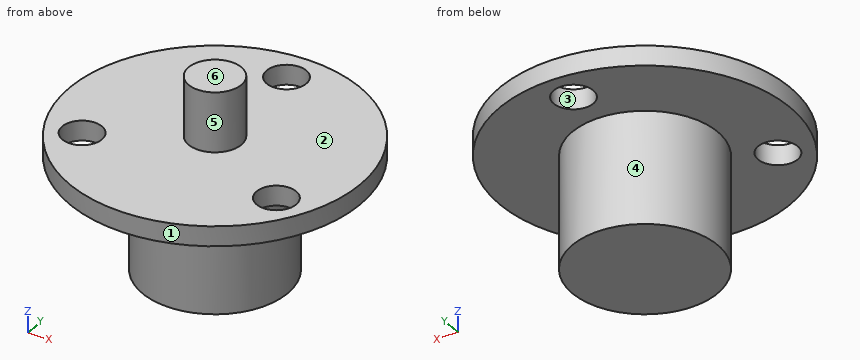
from build123d import *

# Parameters (mm, degrees)
ESQUISSE1_R             = 11
BOSS_EXTRU_1_DEPTH      = 17
ESQUISSE2_R             = 22
BOSS_EXTRU_2_DEPTH      = 3
ESQUISSE3_R             = 4
BOSS_EXTRU_3_DEPTH      = 9
ENL_V_MAT_EXTRU_1_REACH = 38.986
ESQUISSE5_R             = 3


with BuildPart() as part:
    # Esquisse1 → Boss.-Extru.1 (new body)
    with BuildSketch(Plane.XY):
        Circle(ESQUISSE1_R)
    extrude(amount=BOSS_EXTRU_1_DEPTH)

    # Esquisse2 → Boss.-Extru.2 (add)
    with BuildSketch(Plane.XY.offset(17)):
        Circle(ESQUISSE2_R)
    extrude(amount=BOSS_EXTRU_2_DEPTH)

    # Esquisse3 → Boss.-Extru.3 (add)
    with BuildSketch(Plane.XY.offset(20)):
        Circle(ESQUISSE3_R)
    extrude(amount=BOSS_EXTRU_3_DEPTH)

    # Esquisse5 → Enlèv. mat.-Extru.1 (cut, up to next)
    with BuildSketch(Plane.XY.offset(20), mode=Mode.PRIVATE) as enl_v_mat_extru_1_sk1:
        with Locations((0, 17)):
            Circle(ESQUISSE5_R)
    enl_v_mat_extru_1_tool1 = extrude(enl_v_mat_extru_1_sk1.sketch, amount=-ENL_V_MAT_EXTRU_1_REACH, mode=Mode.PRIVATE) & part.part
    # Esquisse5 → Enlèv. mat.-Extru.1 (cut, up to next)
    with BuildSketch(Plane.XY.offset(20), mode=Mode.PRIVATE) as enl_v_mat_extru_1_sk2:
        with Locations((14.722431864, -8.5)):
            Circle(ESQUISSE5_R)
    enl_v_mat_extru_1_tool2 = extrude(enl_v_mat_extru_1_sk2.sketch, amount=-ENL_V_MAT_EXTRU_1_REACH, mode=Mode.PRIVATE) & part.part
    # Esquisse5 → Enlèv. mat.-Extru.1 (cut, up to next)
    with BuildSketch(Plane.XY.offset(20), mode=Mode.PRIVATE) as enl_v_mat_extru_1_sk3:
        with Locations((-14.722431864, -8.5)):
            Circle(ESQUISSE5_R)
    enl_v_mat_extru_1_tool3 = extrude(enl_v_mat_extru_1_sk3.sketch, amount=-ENL_V_MAT_EXTRU_1_REACH, mode=Mode.PRIVATE) & part.part
    add(enl_v_mat_extru_1_tool1.solids().sort_by_distance((0, 17, 20))[0], mode=Mode.SUBTRACT)
    add(enl_v_mat_extru_1_tool2.solids().sort_by_distance((14.722432, -8.5, 20))[0], mode=Mode.SUBTRACT)
    add(enl_v_mat_extru_1_tool3.solids().sort_by_distance((-14.722432, -8.5, 20))[0], mode=Mode.SUBTRACT)


solid = part.part
Source: CAD feature listing. Evaluate the final solid. Frame: model axes, mm. Face numbers are marked on the shaded views. A direction names the side the tool comes from. Round coordinates to 2 decimals unless told otherwise and drop trailing zeros. Loops run counter-clockwise (first coordinate to the right, second up) from the corner with the lowest first, then second, coordinate; pieces in that order, holes last.
Q1. First-contact query: P1, Ø12, axis at x = -15.5, y = 0.5, coming from the -Z side; P2, Ø1.5, axis at x = 1.5, z = 20.5, coming from the +Y side; P3, Ø4, axis at y = 7, z = 12.5, coming from the +X side; P4, Ø1, axis at y = -3.5, z = 24, coming from the +X side. Flat tips, straight axial feed; report the tip coordinate or a pass-through.
Q2. Mould query, pull axis Y, two halves, no side actions, for the marked faces 1, 2 and 3. Classes: pulls with the +Y half, pulls with the -Y half, needs draft (parallel to the pull), parting line crosses it, or undercut.
Q3. Section A-A, the plane y = 17. Return loops of the section in (x, z), plus the area to 3 significant figures.
Q4. Section B-B, the plane x = 0. Return loops of the section in (y, z), plus the area to 3 significant figures.
Q5. Access query for the marked faces 4, 5 and 6. Directions: +Z, -Z, +X, -X, +Y, -Y. A direction counts if a zero-diameter tool reaches every point of the face in a straight line with its end or side. Return the directions, or none.
Q6. Ray query, line 1 (Y direction, x = 0, z = 18.75); line 2 (Z direction, x = 9.5, y = -5); line 3 (Z direction, x = 10.5, y = 11.5). Return the intervals inside material, ascending.
Q7. Section D-D, the plane y = 0. Return loops of the section in (x, z).
Q8. Section C-C, the plane z = 18. Return loops of the section in (x, y), plus the area to 3 significant figures.
Solutions:
1. P1: stops at z = 0
1. P2: stops at y = 21.98
1. P3: stops at x = 9.8
1. P4: stops at x = 2.65
2. face 1: parting line crosses it
2. face 2: needs draft
2. face 3: undercut
3. outline: (-13.96, 17) - (-3, 17) - (-3, 20) - (-13.96, 20) - close; (3, 17) - (13.96, 17) - (13.96, 20) - (3, 20) - close
3. area: 65.8 mm2
4. outline: (-22, 17) - (-11, 17) - (-11, 0) - (11, 0) - (11, 17) - (14, 17) - (14, 20) - (4, 20) - (4, 29) - (-4, 29) - (-4, 20) - (-22, 20) - close; (20, 17) - (22, 17) - (22, 20) - (20, 20) - close
4. area: 560 mm2
5. face 4: -Z
5. face 5: +Z
5. face 6: +Z, +X, -X, +Y, -Y
6. line 1: y = -22 to 14, 20 to 22
6. line 2: z = 0 to 20
6. line 3: z = 17 to 20
7. outline: (-22, 17) - (-11, 17) - (-11, 0) - (11, 0) - (11, 17) - (22, 17) - (22, 20) - (4, 20) - (4, 29) - (-4, 29) - (-4, 20) - (-22, 20) - close
8. outline: circle Ø44 at (0, 0); hole circle Ø6 at (-14.72, -8.5); hole circle Ø6 at (0, 17); hole circle Ø6 at (14.72, -8.5)
8. area: 1,440 mm2
